Geometry check sheet. Reference: the model listing, model coordinates, mm. A direction names the side the tool comes from. Round coordinates to 2 decimals unless told otherwise and drop trailing zeros. Order: outer loops, then holes, each group sorted by start corner. A loop starts at its lowest first (then second) coordinate and runs counter-clockwise, first axis right, second up.
(1) Sectioned sample at B-B (z = 0). Record the boundary of the cut face in (x, y), plus the area to 3 significant figures.
(2) Sectioned sample at C-C (y = 3.5). Record the boundary of the cut face in (x, z), plus the area to 3 significant figures.
(3) Set-up check for faces 1 (the face through (-135.49, 9.13, -35.72)), 2 (the face through (-4, 9, 90)): record each of +Z, -Z, +X, -X, +Y, -Y from which the full face is reachable in a straight line by a thin tool's end or side.
(4) Release check for a two-part mould opening along Z. For faces 3 (the face through (2, 9, -40)), 4 (the face through (297, 9, 1)), 5 (the face through (-4, 9, -90)), 6 (the face through (140, 9, 0)) record: +Z half, -Z half, draft (parallel to the pull), parting line (faces both ways), or undercut.
(5) Sectioned sample at A-A (x = 200). Record the boundary of the cut face in (y, z).
(6) Material ranges on line 1 along X through (y, z) = (6, 0); line 2 along X through (y, z) = (8.25, 23); line 3 along Z through (x, y) = (58.5, 1.5), recorded low to high.
(7) Sectioned sample at D-D (x = 96). Record the boundary of the cut face in (y, z), plus the area to 3 significant figures.
from build123d import *

# Parameters (mm, degrees)
SKETCH1_W           = 594
SKETCH1_H           = 180
BOSS_EXTRUDE1_DEPTH = 18
SKETCH2_R           = 6
CUT_EXTRUDE1_DEPTH  = 40


with BuildPart() as part:
    # Sketch1 → Boss-Extrude1 (new body)
    with BuildSketch(Plane(origin=(0, 0, 0), x_dir=(1, 0, 0), z_dir=(0, 1, 0))):
        Rectangle(SKETCH1_W, SKETCH1_H)
    extrude(amount=BOSS_EXTRUDE1_DEPTH)

    # Sketch2 → Cut-Extrude1 (cut)
    with BuildSketch(Plane(origin=(0, 18, 0), x_dir=(1, 0, 0), z_dir=(0, 1, 0))):
        with Locations((-200, 0)):
            Circle(SKETCH2_R)
        with Locations((200, 0)):
            Circle(SKETCH2_R)
        with BuildLine():
            Line((-125, -40), (125, -40))
            ThreePointArc((125, -40), (135.606601718, -35.606601718), (140, -25))
            Line((140, -25), (140, 25))
            ThreePointArc((140, 25), (135.606601718, 35.606601718), (125, 40))
            Line((125, 40), (-125, 40))
            ThreePointArc((-125, 40), (-135.606601718, 35.606601718), (-140, 25))
            Line((-140, 25), (-140, -25))
            ThreePointArc((-140, -25), (-135.606601718, -35.606601718), (-125, -40))
        make_face()
    extrude(amount=-CUT_EXTRUDE1_DEPTH, mode=Mode.SUBTRACT)


solid = part.part
Answer below:
1. outline: (-297, 0) - (-206, 0) - (-206, 18) - (-297, 18) - close; (-194, 0) - (-140, 0) - (-140, 18) - (-194, 18) - close; (140, 0) - (194, 0) - (194, 18) - (140, 18) - close; (206, 0) - (297, 0) - (297, 18) - (206, 18) - close
1. area: 5,220 mm2
2. outline: (-297, -90) - (297, -90) - (297, 90) - (-297, 90) - close; hole circle Ø12 at (-200, 0); hole (-140, -25) arc R15 ccw to (-125, -40) - (125, -40) arc R15 ccw to (140, -25) - (140, 25) arc R15 ccw to (125, 40) - (-125, 40) arc R15 ccw to (-140, 25) - close; hole circle Ø12 at (200, 0)
2. area: 84,500 mm2
3. face 1: +Y, -Y
3. face 2: +Z, +X, -X, +Y, -Y
4. face 3: undercut
4. face 4: draft
4. face 5: -Z half
4. face 6: undercut
5. outline: (0, -90) - (18, -90) - (18, -6) - (0, -6) - close; (0, 6) - (18, 6) - (18, 90) - (0, 90) - close
6. line 1: x = -297 to -206, -194 to -140, 140 to 194, 206 to 297
6. line 2: x = -297 to -140, 140 to 297
6. line 3: z = -90 to -40, 40 to 90
7. outline: (0, -90) - (18, -90) - (18, -40) - (0, -40) - close; (0, 40) - (18, 40) - (18, 90) - (0, 90) - close
7. area: 1,800 mm2
